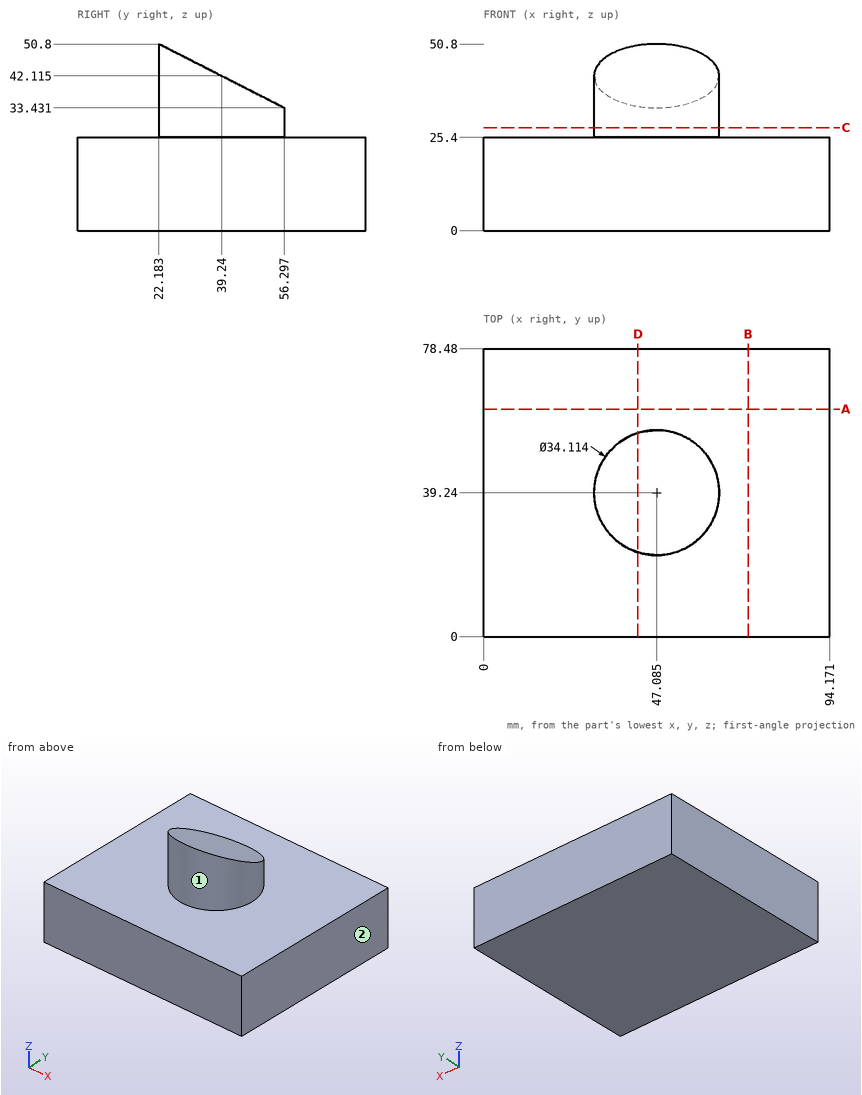
Study the drawing (mm; zero at the part's minimum x, y, z) and answer. A direction names the side the tool comes from. Coordinates: 2 decimals unless noted, no trailing zeros. Write each loop counter-clockwise with the first axis right and the second up, starting at its lowest first coordinate (ties: lowest second). Pieces come first, ordered by that corner, then holes. Notation, with made-up numbers: (-39.75, 88) - (14.25, 88) arc R10 cw to (14.25, 98) - close; hole circle Ø10 at (48, 27.25). An arc over 180 degrees is marked (long way). Answer as a JSON object with one key per item and string values.
Q1. Find section D-D (x = 42). Write down the section's boundary in (y, z) (1 decimal).
Results list:
{"outline": "(0, 0) - (78.5, 0) - (78.5, 25.4) - (55.5, 25.4) - (55.5, 33.8) - (23, 50.4) - (23, 25.4) - (0, 25.4) - close"}
Q2. Find section A-A (y = 62). Write down the section's boundary in (x, z), plus the area to 3 significant figures.
Results list:
{"outline": "(0, 0) - (94.17, 0) - (94.17, 25.4) - (0, 25.4) - close", "area": "2,390 mm^2"}
Q3. Which of the six approach directions +Z, -Z, +X, -X, +Y, -Y give full straight-line access (tool end or side, diameter ignored) to the marked faces 1 and 2?
Results list:
{"face 1": "+Z", "face 2": "+Z, -Z, +X, +Y, -Y"}
Q4. Find section B-B (x = 72). Write down the section's boundary in (y, z).
Results list:
{"outline": "(0, 0) - (78.48, 0) - (78.48, 25.4) - (0, 25.4) - close"}
Q5. Consider L1, parallel to Z at x = 73.5, y = 15; L2, parallel to Y at x = 44.5, z = 46.5 (1 decimal); L3, parallel to X at y = 50, z = 36.5. Determine where each line is inside the solid, lowest interval first. Write a range as from..to.
Results list:
{"L1": "z = 0..25.4", "L2": "y = 22.4..30.6", "L3": "x = 33.85..60.32"}
Q6. Given pin 1 Ø1 at (x, y) = (28.5, 28) entering from +Z, flat-ended and moving along its own axis, determine where the tip first touches the part or whether it passes through.
Results list:
{"pin 1": "stops at z = 25.4"}
Q7. Find section C-C (z = 28). Write down the section's boundary in (x, y) (1 decimal), plus the area to 3 significant figures.
Results list:
{"outline": "circle Ø34.1 at (47.1, 39.2)", "area": "914 mm^2"}
